The drawing under review shows one solid part. Ordinate dimensions are in mm from its lowest x, y, z. Coordinates: 2 decimals unless noted, no trailing zeros. Write each loop counter-clockwise with the first axis right and the second up, starting at its lowest first coordinate (ties: lowest second). Pieces come first, ordered by that corner, then holes.
Q1. To check wall thickness, follow probe 1 along Y at (x, z) = (1.15, 4); probe 2 along Y at (x, z) = (2.6, 51.5); probe 3 along Z at (x, y) = (1.2, 28.5). State the ranges of each line that lie inside material, in increasing order.
Q2. Add section C-C, the plane y = 26. Give the boundary of the cut face in (x, z), plus the area to 3 significant figures.
Q3. Add section B-B, the plane x = 0.5. Give the boundary of the cut face in (y, z), plus the area to 3 significant figures.
Q4. Clearance check with a flat-ended pin moving along its axis: pin 1 Ø1 at (x, y) = (1, 17.5) entering from -Z. State where the tip first meets the part, or that it passes through.
Q5. Add section A-A, the plane z = 47. Give the boundary of the cut face in (x, y), plus the area to 3 significant figures.
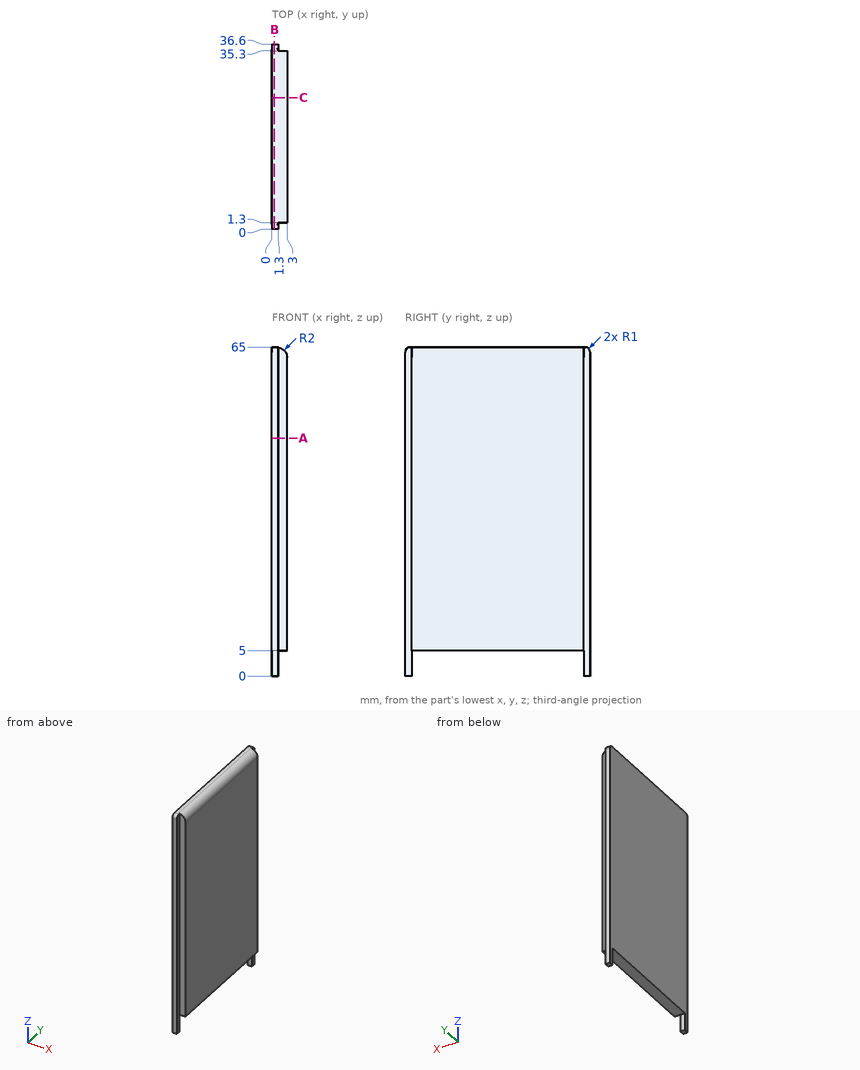
Here are the results:
1. probe 1: y = 0 to 1.3, 35.3 to 36.6
1. probe 2: y = 1.3 to 35.3
1. probe 3: z = 5 to 64.99
2. outline: (0, 5) - (3, 5) - (3, 63) arc R2 ccw to (1, 65) - (0, 65) - close
2. area: 179 mm2
3. outline: (0, 0) - (1.3, 0) - (1.3, 5) - (35.3, 5) - (35.3, 0) - (36.6, 0) - (36.6, 64) arc R1 ccw to (35.6, 65) - (1, 65) arc R1 ccw to (0, 64) - close
3. area: 2,210 mm2
4. pin 1: stops at z = 5
5. outline: (0, 0) - (1.3, 0) - (1.3, 1.3) - (3, 1.3) - (3, 35.3) - (1.3, 35.3) - (1.3, 36.6) - (0, 36.6) - close
5. area: 105 mm2
